```python
from build123d import *

# Parameters (mm, degrees)
F1_DEPTH = 25.4
F2_W     = 7.6199993491
F2_H     = 34.71333161
F2_W_2   = 8.7488871068
F2_H_2   = 34.4311110675
F3_DEPTH = 25.4
F4_DEPTH = 25.4
F5_DEPTH = 25.4


with BuildPart() as f1:
    # F0 (on Right) → F1 (new body)
    with BuildSketch(Plane.YZ):
        with BuildLine():
            ThreePointArc((4.0102475369, 31.2737714921), (13.9789110295, 37.5583620793), (17.8654682829, 48.683334142))
            ThreePointArc((17.8654682829, 48.683334142), (-11.1249720627, 62.6622451715), (-4.0102475369, 31.2737714921))
            Line((-4.0102475369, 31.2737714921), (4.0102475369, 31.2737714921))
        make_face()
        with BuildLine():
            Line((4.0102475369, 31.2737714921), (-4.0102475369, 31.2737714921))
            ThreePointArc((-4.0102475369, 31.2737714921), (0, 30.8178658591), (4.0102475369, 31.2737714921))
        make_face()
        with BuildLine():
            ThreePointArc((4.0102475369, 31.2737714921), (0, 30.8178658591), (-4.0102475369, 31.2737714921))
            Line((-4.0102475369, 31.2737714921), (-4.0102475369, 0))
            Line((-4.0102475369, 0), (4.0922206827, 0))
            Line((4.0922206827, 0), (4.0922206827, 31.2737714921))
            Line((4.0922206827, 31.2737714921), (4.0102475369, 31.2737714921))
        make_face()
        with BuildLine():
            Line((4.0922206827, 0), (-4.0102475369, 0))
            Line((-4.0102475369, 0), (-27.6950067122, -23.4025270809))
            ThreePointArc((-27.6950067122, -23.4025270809), (-24.2033996069, -26.6378410284), (-21.7180567466, -30.6976005513))
            Line((-21.7180567466, -30.6976005513), (0, -8.3255562931))
            Line((0, -8.3255562931), (22.0484417187, -25.4207379206))
            ThreePointArc((22.0484417187, -25.4207379206), (25.5051095185, -22.3833397186), (29.6382622048, -20.3606215012))
            Line((29.6382622048, -20.3606215012), (4.0922206827, 0))
        make_face()
        with BuildLine():
            ThreePointArc((-21.7180567466, -30.6976005513), (-24.2033996069, -26.6378410284), (-27.6950067122, -23.4025270809))
            ThreePointArc((-27.6950067122, -23.4025270809), (-53.1240683212, -45.7241699015), (-20.2587280311, -37.6766659319))
            ThreePointArc((-20.2587280311, -37.6766659319), (-20.6274632454, -34.11166264), (-21.7180567466, -30.6976005513))
        make_face()
        with BuildLine():
            ThreePointArc((52.4996409272, -36.8300005794), (45.2856622606, -22.7420351096), (29.6382622048, -20.3606215012))
            ThreePointArc((29.6382622048, -20.3606215012), (25.5051095185, -22.3833397186), (22.0484417187, -25.4207379206))
            ThreePointArc((22.0484417187, -25.4207379206), (29.0447706115, -53.0892041857), (52.4996409272, -36.8300005794))
        make_face()
    extrude(amount=F1_DEPTH)

    # F2 (on Front) → F3 (cut)
    with BuildSketch(Plane.XZ):
        with Locations((12.6999989152, 48.5422220081)):
            Rectangle(F2_W, F2_H)
        with Locations((12.4177793041, -37.958888337)):
            Rectangle(F2_W_2, F2_H_2)
    extrude(amount=-F3_DEPTH, mode=Mode.SUBTRACT)

    # F2 (on Front) → F4 (cut)
    with BuildSketch(Plane.XZ):
        with Locations((12.6999989152, 48.5422220081)):
            Rectangle(F2_W, F2_H)
        with Locations((12.4177793041, -37.958888337)):
            Rectangle(F2_W_2, F2_H_2)
    extrude(amount=-F4_DEPTH, mode=Mode.SUBTRACT)

    # F2 (on Front) → F5 (cut)
    with BuildSketch(Plane.XZ):
        with Locations((12.6999989152, 48.5422220081)):
            Rectangle(F2_W, F2_H)
        with Locations((12.4177793041, -37.958888337)):
            Rectangle(F2_W_2, F2_H_2)
    extrude(amount=-F5_DEPTH, mode=Mode.SUBTRACT)


solid = f1.part
```
CAD build for the part. Positions are in the model's coordinates, mm. A direction names the side the tool comes from. Round coordinates to 2 decimals unless told otherwise and drop trailing zeros. Write each loop counter-clockwise with the first axis right and the second up, starting at its lowest first coordinate (ties: lowest second). Pieces come first, ordered by that corner, then holes. Notation, with made-up numbers: (1, -30) -> (32, -30) arc R15 cw to (32, -5) -> close; hole circle Ø3 at (-36, -15.75). An arc over 180 degrees is marked (long way). Answer in a Markdown table with one row per item. Add a question column.
Item 1: Saw through at C-C, the plane z = -28.5. Write the cut outline in (x, y).
Item 2: Saw through at A-A, the plane x = 6.5. Write the cut outline in (y, z) (3 decimals).
Item 3: Drill centre lines: line 1 (X direction, y = 22, z = -45.5); line 2 (Y direction, x = 14.25, z = 23.5); line 3 (Z direction, x = 22.75, y = 21.5). Where is each one in solid material? Low to high. Write a range as from..to.
Item 4: Mould opens along X. For faces 4 (the face through (12, 25.4, -36)), 5 (the face through (12.522, 10.87, -16.753)), 6 (the face through (0, -2, -8)) say: pulls with the +X half, pulls with the -X half, needs draft (parallel to the pull), parting line crosses it, or undercut.
Item 5: Saw through at B-B, the plane y = 6.5. Write the cut outline in (x, z).
Item 6: Drop flat-ended pins along their axis: pin 1 Ø2.5 at (x, z) = (14, 55) entering from +Y; pin 2 Ø2.5 at (x, z) = (12, -32) entering from -Y; pin 3 Ø3 at (x, z) = (10.5, 16.5) entering from -Y. Give the stop position or say it passes through.
Item 7: Saw through at D-D, the plane y = -5.5. Write the cut outline in (x, z).
Item 8: Which spindle directions (+Z, -Z, +X, -X, +Y, -Y) get a long thin tool onto all of the face, cutting with end or side? Do faces 1 (the face through (13, 4.092, 15)), 2 (the face through (8.89, 7, 48)), 3 (the face through (8.043, 22, -36)). Say none if no direction does.
Findings below:
| question | item | result |
|---|---|---|
| 1 | outline | (0, -52.48) -> (25.4, -52.48) -> (25.4, -19.58) -> (0, -19.58) -> close; (0, 19.9) -> (8.04, 19.9) -> (8.04, 25.4) -> (16.79, 25.4) -> (16.79, 19.9) -> (25.4, 19.9) -> (25.4, 50.37) -> (0, 50.37) -> close |
| 2 | outline | (-27.695, -23.403) arc R17.418 ccw (long way) to (-21.718, -30.698) -> (0, -8.326) -> (22.048, -25.421) arc R17.363 ccw (long way) to (29.638, -20.361) -> (4.092, 0) -> (4.092, 31.274) -> (4.01, 31.274) arc R17.865 ccw (long way) to (-4.01, 31.274) -> (-4.01, 0) -> close |
| 3 | line 1 | x = 0..8.04, 16.79..25.4 |
| 3 | line 2 | y = -4.01..4.09 |
| 3 | line 3 | z = -47.58..-26.08, -25..-13.87 |
| 4 | face 4 | undercut |
| 4 | face 5 | needs draft |
| 4 | face 6 | pulls with the -X half |
| 5 | outline | (0, -13.37) -> (25.4, -13.37) -> (25.4, -1.92) -> (0, -1.92) -> close; (0, 32.04) -> (8.89, 32.04) -> (8.89, 65.32) -> (0, 65.32) -> close; (16.51, 32.04) -> (25.4, 32.04) -> (25.4, 65.32) -> (16.51, 65.32) -> close |
| 6 | pin 1 | stops at y = 0 |
| 6 | pin 2 | stops at y = -54.52 |
| 6 | pin 3 | stops at y = -4.01 |
| 7 | outline | (0, -13.99) -> (25.4, -13.99) -> (25.4, -1.47) -> (0, -1.47) -> close; (0, 31.69) -> (25.4, 31.69) -> (25.4, 65.68) -> (0, 65.68) -> close |
| 8 | face 1 | +X, -X, +Y |
| 8 | face 2 | +Y |
| 8 | face 3 | -Z |
